from build123d import *

# Parameters (mm, degrees)
SKETCH1_R           = 35
BOSS_EXTRUDE1_DEPTH = 4
SKETCH2_R           = 3.5
SKETCH2_W           = 20
SKETCH2_H           = 40
CUT_EXTRUDE1_DEPTH  = 5


with BuildPart() as part:
    # Sketch1 → Boss-Extrude1 (new body)
    with BuildSketch(Plane(origin=(0, 0, 0), x_dir=(1, 0, 0), z_dir=(0, 1, 0))):
        with Locations(Location((0, 0, 0), (0, 0, 270))):
            Circle(SKETCH1_R)
    extrude(amount=BOSS_EXTRUDE1_DEPTH)

    # Sketch2 → Cut-Extrude1 (cut)
    with BuildSketch(Plane(origin=(0, 0, 0), x_dir=(1, 0, 0), z_dir=(0, 1, 0))):
        with Locations(Location((-4.5, 25, 0), (0, 0, 270))):
            Circle(SKETCH2_R)
        with Locations(Location((4.5, 25, 0), (0, 0, 90))):
            Circle(SKETCH2_R)
        with Locations(Location((4.5, -25, 0), (0, 0, 270))):
            Circle(SKETCH2_R)
        with Locations(Location((-4.5, -25, 0), (0, 0, 90))):
            Circle(SKETCH2_R)
        with Locations(Location((-28.346706054, 0, 0), (0, 0, 270))):
            Circle(SKETCH2_R)
        with Locations(Location((28.346706054, 0, 0), (0, 0, 90))):
            Circle(SKETCH2_R)
        Rectangle(SKETCH2_W, SKETCH2_H)
        with BuildLine():
            Line((-17, 20), (-17, -20))
            ThreePointArc((-17, -20), (-20, -23), (-23, -20))
            Line((-23, -20), (-23, 20))
            ThreePointArc((-23, 20), (-20, 23), (-17, 20))
        make_face()
        with BuildLine():
            Line((17, 20), (17, -20))
            ThreePointArc((17, -20), (20, -23), (23, -20))
            Line((23, -20), (23, 20))
            ThreePointArc((23, 20), (20, 23), (17, 20))
        make_face()
    extrude(amount=CUT_EXTRUDE1_DEPTH, mode=Mode.SUBTRACT)


solid = part.part
CAD build for the part. Positions are in the model's coordinates, mm. A direction names the side the tool comes from. Give positions to 0.01 mm unless a question says otherwise; leave off trailing zeros. Write each loop counter-clockwise with the first axis right and the second up, starting at its lowest first coordinate (ties: lowest second). Pieces come first, ordered by that corner, then holes. Notation, with made-up numbers: (10, -23) -> (67, -23) arc R19 ccw to (67, 0) -> close; hole circle Ø4 at (33, -23.75). An arc over 180 degrees is marked (long way). Return JSON: item names as keys, results as strings.
Item 1: Band-saw the part on A-A (x = 0). List the corners of the cut face in (y, z).
Answer below:
{"outline": "(0, -35) -> (4, -35) -> (4, -20) -> (0, -20) -> close; (0, 20) -> (4, 20) -> (4, 35) -> (0, 35) -> close"}
Item 2: Two-plate mould, pull along X, no slides. Class faces 3 (the cylindrical face through (-21, 2, -28)), 4 (the cylindrical face through (20, 2, 23)), 5 (the flat face through (16, 0, 0)): +X half, -X half, draft (parallel to the pull), parting line (faces both ways), or undercut.
Answer below:
{"face 3": "parting line", "face 4": "undercut", "face 5": "draft"}
Item 3: Band-saw the part on B-B (z = 0). List the corners of the cut face in (x, y), then the cut area to 3 significant figures.
Answer below:
{"outline": "(-35, 0) -> (-31.85, 0) -> (-31.85, 4) -> (-35, 4) -> close; (-24.85, 0) -> (-23, 0) -> (-23, 4) -> (-24.85, 4) -> close; (-17, 0) -> (-10, 0) -> (-10, 4) -> (-17, 4) -> close; (10, 0) -> (17, 0) -> (17, 4) -> (10, 4) -> close; (23, 0) -> (24.85, 0) -> (24.85, 4) -> (23, 4) -> close; (31.85, 0) -> (35, 0) -> (35, 4) -> (31.85, 4) -> close", "area": "96.0 mm2"}
Item 4: Band-saw the part on D-D (z = -25). List the corners of the cut face in (x, y).
Answer below:
{"outline": "(-24.49, 0) -> (-8, 0) -> (-8, 4) -> (-24.49, 4) -> close; (-1, 0) -> (1, 0) -> (1, 4) -> (-1, 4) -> close; (8, 0) -> (24.49, 0) -> (24.49, 4) -> (8, 4) -> close"}
Item 5: Drop flat-ended pins along their axis: pin 1 (1.2 mm diameter, centred on y = 2, z = 7, fed in from +X); pin 2 (1.5 mm diameter, centred on x = -14.5, y = 1, fed in from +Z); pin 3 (5 mm diameter, centred on x = 2.5, z = 15.5, fed in from -Y) (3 decimals); pin 4 (2 mm diameter, centred on y = 1, z = 1.5, fed in from -X). Give the stop position or say it passes through.
Answer below:
{"pin 1": "stops at x = 34.41", "pin 2": "stops at z = 32.19", "pin 3": "passes through", "pin 4": "stops at x = -35"}
Item 6: Band-saw the part on C-C (y = 0.75). Give the number of separate pieces and of enclosed holes in the cut face, then the cut area to 3 significant figures.
Answer below:
{"separate pieces": "1", "enclosed holes": "9", "area": "2,280 mm2"}
Item 7: Tool access for faces 1 (the flat face through (-17, 2, 0)), 2 (the flat face through (16, 4, 0)): list every direction of +Z, -Z, +X, -X, +Y, -Y with a clear straight run to the whole face (end or side of a thin tool).
Answer below:
{"face 1": "+Y, -Y", "face 2": "+Z, -Z, +X, -X, +Y"}
Item 8: Drill centre lines: probe 1 along Z at (x, y) = (5, 2.1); probe 2 along Z at (x, y) = (2, 2.7); probe 3 along X at (y, z) = (1.1, -3). Where is each one in solid material? Low to high.
Answer below:
{"probe 1": "z = -34.64 to -28.46, -21.54 to -20, 20 to 21.54, 28.46 to 34.64", "probe 2": "z = -34.94 to -27.45, -22.55 to -20, 20 to 22.55, 27.45 to 34.94", "probe 3": "x = -34.87 to -30.15, -26.54 to -23, -17 to -10, 10 to 17, 23 to 26.54, 30.15 to 34.87"}
